Model file for the job. Use its own axes, mm. Face numbers are marked on the shaded views. A direction names the side the tool comes from. Round coordinates to 2 decimals unless told otherwise and drop trailing zeros. Order: outer loops, then holes, each group sorted by start corner. A loop starts at its lowest first (then second) coordinate and runs counter-clockwise, first axis right, second up. Notation, with made-up numbers: (59, -2.75) -> (107, -2.75) arc R10 cw to (107, 8.25) -> close; hole circle Ø6 at (73, 68). An arc over 180 degrees is marked (long way). Use CSV: the item, a comma, the result in double quotes.
```python
from build123d import *

# Parameters (mm, degrees)
SKETCH_1_W          = 30
SKETCH_1_H          = 35
SKETCH_1_R          = 1.65
EXTRUDE_1_DEPTH     = 3
SKETCH_2_W          = 20
SKETCH_2_H          = 20
CUT_EXTRUDE_1_DEPTH = 6
SKETCH_3_W          = 3
SKETCH_3_H          = 15
EXTRUDE_2_DEPTH     = 6
SKETCH_4_W          = 48
SKETCH_4_H          = 24
EXTRUDE_3_DEPTH     = 3
SKETCH_6_R          = 0.75
CUT_EXTRUDE_2_DEPTH = 5


with BuildPart() as part:
    # 草图1 → 凸台-拉伸1 (new body)
    with BuildSketch(Plane.XY):
        with Locations((5.815384615, -13.146153846)):
            Rectangle(SKETCH_1_W, SKETCH_1_H)
        with Locations((0.815384615, -3.646153846)):
            Circle(SKETCH_1_R, mode=Mode.SUBTRACT)
        with Locations((10.815384615, -3.646153846)):
            Circle(SKETCH_1_R, mode=Mode.SUBTRACT)
    extrude(amount=EXTRUDE_1_DEPTH)

    # 草图2 → 切除-拉伸1 (cut)
    with BuildSketch(Plane.XY.offset(3)):
        with Locations((5.815384615, -20.646153846)):
            Rectangle(SKETCH_2_W, SKETCH_2_H)
        with BuildLine():
            Line((-9.184615385, -0.646153846), (-9.184615385, 4.353846154))
            Line((-9.184615385, 4.353846154), (-4.184615385, 4.353846154))
            ThreePointArc((-4.184615385, 4.353846154), (-7.720149291, 2.88938006), (-9.184615385, -0.646153846))
        make_face()
        with BuildLine():
            Line((20.815384615, -0.646153846), (20.815384615, 4.353846154))
            Line((20.815384615, 4.353846154), (15.815384615, 4.353846154))
            ThreePointArc((15.815384615, 4.353846154), (19.350918521, 2.88938006), (20.815384615, -0.646153846))
        make_face()
    extrude(amount=-CUT_EXTRUDE_1_DEPTH, mode=Mode.SUBTRACT)

    # 草图3 → 凸台-拉伸2 (add)
    with BuildSketch(Plane.XY.offset(3)):
        with Locations((-5.684615385, -23.146153846)):
            Rectangle(SKETCH_3_W, SKETCH_3_H)
        with Locations((17.315384615, -23.146153846)):
            Rectangle(SKETCH_3_W, SKETCH_3_H)
    extrude(amount=EXTRUDE_2_DEPTH)

    # 草图4 → 凸台-拉伸3 (add)
    with BuildSketch(Plane.XY.offset(9)):
        with Locations((5.815384615, -26.646153846)):
            Rectangle(SKETCH_4_W, SKETCH_4_H)
    extrude(amount=EXTRUDE_3_DEPTH)

    # 草图6 → 切除-拉伸2 (cut)
    with BuildSketch(Plane.XY.offset(12)):
        with Locations((-15.784615385, -17.246153846)):
            Circle(SKETCH_6_R)
        with Locations((-15.784615385, -36.046153846)):
            Circle(SKETCH_6_R)
        with Locations((27.415384615, -36.046153846)):
            Circle(SKETCH_6_R)
        with Locations((27.415384615, -17.246153846)):
            Circle(SKETCH_6_R)
    extrude(amount=-CUT_EXTRUDE_2_DEPTH, mode=Mode.SUBTRACT)


solid = part.part
```
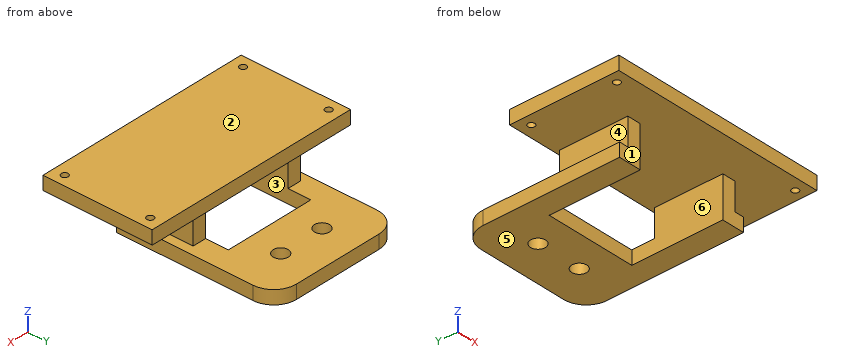
Q1. Mould opens along X. For the marked faces 4, 5 and 6 say: +X half, -X half, draft (parallel to the pull), parting line (faces both ways), or undercut.
From the geometry:
face 4,"-X half"
face 5,"draft"
face 6,"undercut"
Q2. Which spindle directions (+Z, -Z, +X, -X, +Y, -Y) get a long thin tool onto all of the face, cutting with end or side? Do the marked faces 1, 2 and 3. Say none if no direction does.
From the geometry:
face 1,"-Z, +X, -X, -Y"
face 2,"+Z, +X, -X, +Y, -Y"
face 3,"-Z, -Y"
Q3. Cut at D-D (y = -24.5). Give the cut face in (x, z), plus the area to 3 significant figures.
From the geometry:
outline,"(-18.18, 9) -> (-7.18, 9) -> (-7.18, 3) -> (-9.18, 3) -> (-9.18, 0) -> (-4.18, 0) -> (-4.18, 9) -> (15.82, 9) -> (15.82, 0) -> (20.82, 0) -> (20.82, 3) -> (18.82, 3) -> (18.82, 9) -> (29.82, 9) -> (29.82, 12) -> (-18.18, 12) -> close"
area,"210 mm²"
Q4. Cut at C-C (z = 1.5). Give the cut face in (x, y).
From the geometry:
outline,"(-9.18, -30.65) -> (-4.18, -30.65) -> (-4.18, -10.65) -> (15.82, -10.65) -> (15.82, -30.65) -> (20.82, -30.65) -> (20.82, -0.65) arc R5 ccw to (15.82, 4.35) -> (-4.18, 4.35) arc R5 ccw to (-9.18, -0.65) -> close; hole circle Ø3.3 at (0.82, -3.65); hole circle Ø3.3 at (10.82, -3.65)"
Q5. Probe line 1 along Z through (x, y) = (11, -25); line 2 along X through (y, z) = (-25, 0.75); line 3 along Z through (x, y) = (12.5, 1). List the from-to ranges inside material, lowest first.
From the geometry:
line 1,"z = 9 to 12"
line 2,"x = -9.18 to -4.18, 15.82 to 20.82"
line 3,"z = 0 to 3"
Q6. Cut at B-B (y = -12). Give the cut face in (x, z), plus the area to 3 significant figures.
From the geometry:
outline,"(-9.18, 0) -> (-4.18, 0) -> (-4.18, 3) -> (-9.18, 3) -> close; (15.82, 0) -> (20.82, 0) -> (20.82, 3) -> (15.82, 3) -> close"
area,"30.0 mm²"
Q7. Pin check, flat tips, straight feed: pin 1 (9 mm diameter, centred on x = 12.5, y = -8.5, fed in from +Z); pin 2 (2.5 mm diameter, centred on y = -10.5, z = 1, fed in from +X); pin 3 (5 mm diameter, centred on x = 3, z = 2, fed in from -Y); pin 4 (6.5 mm diameter, centred on y = -26.5, z = 6.5, fed in from -X). Stop position of each tip, or through.
From the geometry:
pin 1,"stops at z = 3"
pin 2,"stops at x = 20.82"
pin 3,"stops at y = -10.65"
pin 4,"stops at x = -18.18"
Q8. Cut at A-A (x = -2). Give the cut face in (y, z), plus the area to 3 significant figures.
From the geometry:
outline,"(-38.65, 9) -> (-14.65, 9) -> (-14.65, 12) -> (-38.65, 12) -> close; (-10.65, 0) -> (4.35, 0) -> (4.35, 3) -> (-10.65, 3) -> close"
area,"117 mm²"
